Autodesk Inventor part; units mm, degrees
ref_plane "YZ Plane" through (0, 0, 0) normal (1, 0, 0) x (0, 1, 0)
ref_plane "XZ Plane" through (0, 0, 0) normal (0, 1, 0) x (-1, 0, 0)
ref_plane "XY Plane" through (0, 0, 0) normal (0, 0, 1) x (1, 0, 0)
sketch "Sketch1" plane through (0, 0, 0) normal (0, 1, 0) x (-1, 0, 0)
  line L0 (0, 0) -> (-30.6, 0)
  line L1 (0, 0) -> (30.6, 0)
  line L2 (30.6, 0) -> (41.764, -19.3366)
  line L3 (30.6, 0) -> (52.928, 0) construction
  line L4 (-30.6, 0) -> (-41.764, -19.3366)
  line L5 (-30.6, 0) -> (-8.272, 0) construction
  line L6 (0, 0) -> (0, 77)
  line L7 (0, 0) -> (0, -3)
  line L8 (-35.3569, -8.2392) -> (-32.7588, -9.7392)
  line L9 (35.0582, -7.7219) -> (32.4602, -9.2219)
  line L10 (32.4602, -9.2219) -> (28.8679, -3)
  line L11 (28.8679, -3) -> (0, -3)
  line L12 (0, -3) -> (-28.8679, -3)
  line L13 (-28.8679, -3) -> (-32.7588, -9.7392)
  line L14 (-32.7588, -9.7392) -> (-38.9714, -20.4998)
  line L15 (32.4602, -9.2219) -> (38.9714, -20.4998)
  arc A0 (38.9714, -20.4998) -> (41.764, -19.3366) centre (0, 77) ccw
  arc A1 (-41.764, -19.3366) -> (-38.9714, -20.4998) centre (0, 77) ccw
  dimension "d0" = 30.6
  dimension "d1" = 30.6
  dimension "d2" = 22.328
  dimension "d3" = 60
  dimension "d4" = 22.328
  dimension "d5" = 120
  dimension "d6" = 77
  dimension "d7" = 3
  dimension "d8" = 3
  dimension "d9" = 3
extrude "Extrusion1" add sketch "Sketch1" along normal blind 40
sketch "Sketch2" plane through (0, 0, 0) normal (0, -1, 0) x (1, 0, 0)
  line L0 (0, 0) -> (0, 5)
  circle A0 centre (0, 5) radius 1.5
  line L1 (-41.764, -19.3366) -> (-39.264, -15.0065)
  line L2 (-41.764, -19.3366) -> (-30.6, 0)
  line L3 (-39.264, -15.0065) -> (-43.5941, -12.5065)
  arc A1 (38.9714, -20.4998) -> (41.764, -19.3366) centre (0, 77) ccw
  line L4 (38.9714, -20.4998) -> (39.264, -15.0065)
  line L5 (30.6, 0) -> (41.764, -19.3366)
  line L6 (41.764, -19.3366) -> (39.264, -15.0065)
  line L7 (39.264, -15.0065) -> (43.5941, -12.5065)
  circle A2 centre (43.5941, -12.5065) radius 1.5
  circle A3 centre (-43.5941, -12.5065) radius 1.5
  circle A4 centre (-43.5941, -12.5065) radius 4
  circle A5 centre (0, 5) radius 4
  circle A6 centre (43.5941, -12.5065) radius 4
  line L8 (43.5941, -12.5065) -> (45.5941, -15.9706)
  line L9 (45.5941, -15.9706) -> (41.264, -18.4706)
  line L10 (43.5941, -12.5065) -> (41.5941, -9.0424)
  line L11 (41.5941, -9.0424) -> (37.264, -11.5424)
  line L12 (4, 5) -> (4, 0)
  line L13 (-30.6, 0) -> (30.6, 0)
  line L14 (-4, 5) -> (-4, 0)
  line L15 (-43.5941, -12.5065) -> (-45.5941, -15.9706)
  line L16 (-45.5941, -15.9706) -> (-41.264, -18.4706)
  line L17 (-41.764, -19.3366) -> (-30.6, 0)
  line L18 (-43.5941, -12.5065) -> (-41.5941, -9.0424)
  line L19 (-41.5941, -9.0424) -> (-37.264, -11.5424)
  dimension "d12" = 5
  dimension "d13" = 3
  dimension "d14" = 5
  dimension "d15" = 5
  dimension "d16" = 5.5011
  dimension "d17" = 5
  dimension "d18" = 3
  dimension "d19" = 8
  dimension "d20" = 8
  dimension "d21" = 8
extrude "Extrusion2" add sketch "Sketch2" against normal blind 3 contours L13 L14 A5 L0 | L0 A5 L12 L13 | A5 | L16 A4 L3 L1 | L3 A4 L19 L2 | L15 A3 L3 A4 | A4 L18 A3 L15 | L3 A3 L18 A4 | L15 L3 A3 | A3 L18 L15 | L3 L18 A3 | L7 A6 L9 L5 | L5 L11 A6 L7 | A6 L10 A2 L7 | L7 A2 L8 A6 | L8 A2 L10 A6 | A2 L10 L7 | L7 L8 A2 | L8 L10 A2
sketch "Sketch3" plane through (0, 3, 0) normal (0, 1, 0) x (1, 0, 0)
  arc A0 (41.5941, 9.0424) -> (45.5941, 15.9706) centre (43.5941, 12.5065) ccw
  circle A1 centre (43.5941, 12.5065) radius 1.5
  arc A2 (-45.5941, 15.9706) -> (-41.5941, 9.0424) centre (-43.5941, 12.5065) ccw
  circle A3 centre (-43.5941, 12.5065) radius 1.5
  point P0 (0, 0)
  dimension "d24" = 3
extrude "Extrusion3" cut sketch "Sketch3" against normal blind 3
sketch "Sketch4" plane through (-30.6, 40, 0) normal (0, 0, 1) x (1, 0, 0)
  point P0 (30.6, -40)
sketch "Sketch5" plane through (0, 40, 0) normal (0, 1, 0) x (1, 0, 0)
  circle A0 centre (0, -5) radius 1.5
  line L0 (0, -5) -> (17.465, -5)
  line L1 (0, -5) -> (-17.465, -5)
  circle A1 centre (-17.465, -5) radius 1.75
  circle A2 centre (17.465, -5) radius 1.75
  line L2 (-17.465, -5) -> (-21.465, -5)
  line L3 (-21.465, -5) -> (-21.465, 0)
  line L4 (-17.465, -5) -> (-13.465, -5)
  line L5 (-13.465, -5) -> (-13.465, 0)
  circle A3 centre (-17.465, -5) radius 4
  line L6 (17.465, -5) -> (13.465, -5)
  line L7 (13.465, -5) -> (13.465, 0)
  line L8 (-30.6, 0) -> (30.6, 0)
  line L9 (17.465, -5) -> (21.465, -5)
  line L10 (21.465, -5) -> (21.465, 0)
  circle A4 centre (17.465, -5) radius 4
  point P0 (0, 0)
  dimension "d27" = 17.465
  dimension "d28" = 17.465
  dimension "d29" = 3.5
  dimension "d30" = 4
  dimension "d31" = 4
  dimension "d32" = 4
  dimension "d33" = 4
extrude "Extrusion4" add sketch "Sketch5" against normal blind 3 contours A4 L9 A2 L0 | L7 L8 L10 A4 | L0 A2 L9 A4 | A3 L2 A1 L1 | A3 L3 L8 L5 | L1 A1 L2 A3 | A2 L9 L0 | L1 L2 A1 picked at (18.233, -4.1331) picked at (-16.697, -4.1331)
sketch "Sketch6" plane through (0, 40, 0) normal (0, 1, 0) x (1, 0, 0)
  arc A0 (-19.215, -5) -> (-15.715, -5) centre (-17.465, -5) ccw
  line L0 (-19.215, -5) -> (-15.715, -5)
  circle A1 centre (-17.465, -5) radius 1.75
  arc A2 (15.715, -5) -> (19.215, -5) centre (17.465, -5) ccw
  line L1 (15.715, -5) -> (19.215, -5)
  circle A3 centre (17.465, -5) radius 1.75
  point P0 (0, 0)
extrude "Extrusion5" cut sketch "Sketch6" against normal blind 3 contours A1 L0 | A3 L1
sketch "Sketch7" plane through (0, 3, 0) normal (0, 1, 0) x (1, 0, 0)
  circle A0 centre (0, -5) radius 1.5
  circle A1 centre (0, -5) radius 1.75
  circle A2 centre (43.5941, 12.5065) radius 1.5
  circle A3 centre (43.5941, 12.5065) radius 1.75
  circle A4 centre (-43.5941, 12.5065) radius 1.5
  circle A5 centre (-43.5941, 12.5065) radius 1.75
  point P0 (0, 0)
  dimension "d38" = 3.5
  dimension "d39" = 3.5
  dimension "d40" = 3.5
extrude "Extrusion6" cut sketch "Sketch7" against normal blind 3 contours A1 | A3 | A4 | A5
properties part number "Capcture Zone2"
Verification items for the finished model (mm, model axes). A direction names the side the tool comes from. Give positions to 0.01 mm unless a question says otherwise; leave off trailing zeros. Write each loop counter-clockwise with the first axis right and the second up, starting at its lowest first coordinate (ties: lowest second). Pieces come first, ordered by that corner, then holes. Notation, with made-up numbers: M 38,-14.75 L 58,-14.75 A19 ccw 58,20.25 Z; hole C 14,-7.75 d6. An arc over 180 degrees is marked long. Put each result on its own line as item: value. Start each with the question number.
1. Set-up check for faces 4 (the face through (4, 1, 3)), 5 (the face through (13.465, 39, 3)), 6 (the face through (42, 3, -15)): record each of +Z, -Z, +X, -X, +Y, -Y from which the full face is reachable in a straight line by a thin tool's end or side.
2. Scan lines: line 1 along X through (y, z) = (1.65, 5); line 2 along Z through (x, y) = (0, 2.25); line 3 along Y through (x, z) = (-19.5, 0.25). Record each from-to range of solid material in increasing order. Write a range as [from, to].
3. Section check A-A (x = 0). Record the cut outline in (y, z), and give its area (4 significant figures).
4. Section check C-C (y = 29.5). Record the cut outline in (x, z), and give its area (3 significant figures).
5. Go/stop test with flat-tipped pins: pin 1 Ø8 at (x, z) = (-43, -16) entering from +Y; pin 2 Ø1.5 at (y, z) = (1, 1.5) entering from +X; pin 3 Ø1.5 at (x, y) = (-17, 10.5) entering from +Z; pin 4 Ø2 at (y, z) = (20, -4) entering from +X. Record where each tip stops, or that it passes through.
6. Draft check along Z on faces 1 (the face through (-39.459, 1.479, -10.275)), 2 (the face through (-4, 1, 3)), 3 (the face through (-0.38, 1.52, 6.71)). Enter one of: +Z half, -Z half, draft (parallel to the pull), parting line (faces both ways), or undercut.
7. Section check B-B (z = -17). Record the cut outline in (x, y).
Answer list:
1. face 4: +Z, +X, +Y, -Y
1. face 5: +Z, +Y, -Y
1. face 6: +Z, +X, +Y
2. line 1: [-4, -1.75], [1.75, 4]
2. line 2: [-3, 3.25], [6.75, 9]
2. line 3: [37, 40]
3. outline: M 0,-3 L 40,-3 L 40,0 L 3,0 L 3,3.25 L 0,3.25 Z; M 0,6.75 L 3,6.75 L 3,9 L 0,9 Z
3. area: 136.5 mm2
4. outline: M -41.76,-19.34 A104.8 ccw -38.97,-20.5 L -32.46,-9.22 L -28.87,-3 L 28.87,-3 L 32.76,-9.74 L 38.97,-20.5 A105.2 ccw 41.76,-19.34 L 30.6,0 L -30.6,0 Z
4. area: 306 mm2
5. pin 1: y = 40
5. pin 2: x = 4
5. pin 3: z = 0
5. pin 4: x = 33.49
6. face 1: +Z half
6. face 2: draft
6. face 3: undercut
7. outline: M -43.81,0 L -36.95,0 L -36.95,40 L -40.41,40 L -40.41,3 L -43.81,3 Z; M 36.95,0 L 43.81,0 L 43.81,3 L 40.41,3 L 40.41,40 L 36.95,40 Z
